Autodesk Inventor part; units mm, degrees
ref_plane "YZ Plane" through (0, 0, 0) normal (1, 0, 0) x (0, 1, 0)
ref_plane "XZ Plane" through (0, 0, 0) normal (0, 1, 0) x (-1, 0, 0)
ref_plane "XY Plane" through (0, 0, 0) normal (0, 0, 1) x (1, 0, 0)
sketch "Skizze1" plane through (0, 0, 0) normal (0, 1, 0) x (-1, 0, 0)
  line L0 (10.5, 52.028) -> (10.5, 7.028)
  line L1 (10.5, 7.028) -> (13.5, 7.028)
  line L2 (13.5, 7.028) -> (13.5, -7.028)
  line L3 (13.5, -7.028) -> (10.5, -7.028)
  line L4 (10.5, -7.028) -> (10.5, -40.028)
  line L5 (10.5, -40.028) -> (0, -40.028)
  line L6 (0, 52.028) -> (0, -40.028)
  line L7 (0, 0) -> (13.5, 0) construction
  line L8 (10.5, 52.028) -> (0, 52.028)
  point P0 (12, 7.028)
  dimension "d0" = 14.056
  dimension "d1" = 21
  dimension "d2" = 27
  dimension "d14" = 45
  dimension "d15" = 33
revolve "Umdrehung1" add sketch "Skizze1" angle 360 about axis through (0, 0, 52.028) along (0, 0, -1)
sketch "Skizze2" plane through (0, 0, 52.028) normal (0, 0, 1) x (1, 0, 0)
  point P0 (0, 0)
  point P1 (0, 0)
hole "Bohrung1" at (0, 0, 52.028) direction (0, 0, -1) diameter 18 end through all
properties part number "vernindung"
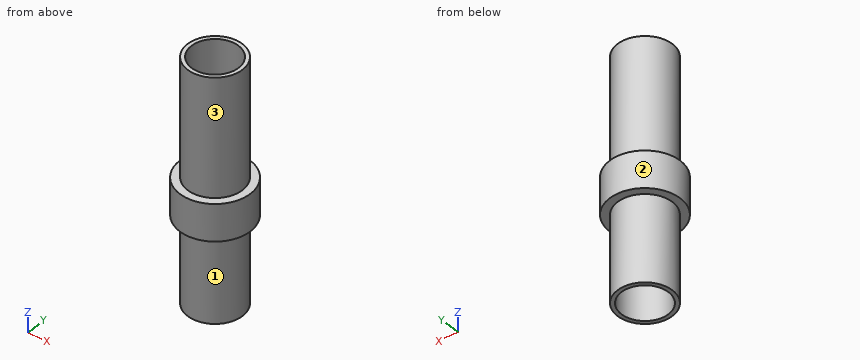
CAD build for the part. Positions are in the model's coordinates, mm. Face numbers are marked on the shaded views. A direction names the side the tool comes from. Round coordinates to 2 decimals unless told otherwise and drop trailing zeros. Order: outer loops, then holes, each group sorted by start corner. A loop starts at its lowest first (then second) coordinate and runs counter-clockwise, first axis right, second up. Notation, with made-up numbers: (43.25, -27.75) -> (76.25, -27.75) arc R27 ccw to (76.25, -8.75) -> close; hole circle Ø8 at (-17.5, 43.25). An arc over 180 degrees is marked (long way). Write each question's results on one line, items separated by ' | '.
1. Cut at D-D (y = 11.5). Give the cut face in (x, z), plus the area to 3 significant figures.
Findings below:
outline: (-7.07, -7.03) -> (7.07, -7.03) -> (7.07, 7.03) -> (-7.07, 7.03) -> close | area: 199 mm²
2. 3-axis set-ups, long thin cutter, end or side, ignore diameter. For the marked faces 1, 2 and 3: which of +Z, -Z, +X, -X, +Y, -Y reach the whole face in a straight line?
Findings below:
face 1: -Z | face 2: +Z, -Z | face 3: +Z
3. Flat gauge pins, fed straight in: P1, Ø8, axis at x = -4, z = -18, coming from the +Y side; P2, Ø12, axis at x = 10.5, z = -5, coming from the +Y side; P3, Ø5, axis at x = 3, y = 4.5, coming from the -Z side; P4, Ø4, axis at x = -9, z = -15, coming from the -Y side. Where does each tip first touch, or does it go through?
Findings below:
P1: stops at y = 10.5 | P2: stops at y = 12.73 | P3: passes through | P4: stops at y = -7.83
4. Cut at C-C (z = 39). Give the cut face in (x, y).
Findings below:
outline: circle Ø21 at (0, 0); hole circle Ø18 at (0, 0)
5. Wall check: line 1 along X through (y, z) = (0.25, 43.5); line 2 along Y through (x, z) = (0, 2.5). Give the ranges that are in metal, low to high. Write a range as [from, to].
Findings below:
line 1: x = [-10.5, -9], [9, 10.5] | line 2: y = [-13.5, -9], [9, 13.5]
6. Cut at A-A (y = 0). Give the cut face in (x, z), plus the area to 3 significant figures.
Findings below:
outline: (-13.5, -7.03) -> (-10.5, -7.03) -> (-10.5, -40.03) -> (-9, -40.03) -> (-9, 52.03) -> (-10.5, 52.03) -> (-10.5, 7.03) -> (-13.5, 7.03) -> close; (9, -40.03) -> (10.5, -40.03) -> (10.5, -7.03) -> (13.5, -7.03) -> (13.5, 7.03) -> (10.5, 7.03) -> (10.5, 52.03) -> (9, 52.03) -> close | area: 361 mm²
